Source: CAD feature listing. Evaluate the final solid. Frame: model axes, mm. A direction names the side the tool comes from. Coordinates: 2 decimals unless noted, no trailing zeros. Write each loop counter-clockwise with the first axis right and the second up, starting at its lowest first coordinate (ties: lowest second). Pieces come first, ordered by that corner, then holes. Notation, with made-up numbers: (11.25, 86.5) -> (25.25, 86.5) arc R9 cw to (25.25, 101.5) -> close; hole circle Ø4 at (46.25, 11). An arc over 180 degrees is marked (long way). Write item = value, one per line.
from build123d import *

# Parameters (mm, degrees)
SKETCH1_W           = 540
SKETCH1_H           = 330
BOSS_EXTRUDE1_DEPTH = 3
SKETCH2_W           = 540
SKETCH2_H           = 330
SKETCH2_W_2         = 500
SKETCH2_H_2         = 290
BOSS_EXTRUDE2_DEPTH = 25
FILLET1_R           = 5
SKETCH4_R           = 1.6
CUT_EXTRUDE1_DEPTH  = 28
SKETCH5_R           = 15
CUT_EXTRUDE2_DEPTH  = 3
SKETCH6_W           = 10
SKETCH6_H           = 290
BOSS_EXTRUDE3_DEPTH = 10
FILLET3_R           = 4
CHAMFER1_SIZE       = 5
SKETCH7_R           = 2.6
CUT_EXTRUDE3_DEPTH  = 3
SKETCH9_R           = 2.6
CUT_EXTRUDE4_DEPTH  = 47
SKETCH11_W          = 8
SKETCH11_H          = 140
BOSS_EXTRUDE4_DEPTH = 66
SKETCH12_R          = 6.1
CUT_EXTRUDE5_DEPTH  = 8
SKETCH13_W          = 8
SKETCH13_H          = 69
SKETCH13_W_2        = 20
SKETCH13_H_2        = 40.75
BOSS_EXTRUDE5_DEPTH = 27
SKETCH15_W          = 8
SKETCH15_H          = 47
CUT_EXTRUDE6_DEPTH  = 66
FILLET4_R           = 4
FILLET5_R           = 10
FILLET6_R           = 5
FILLET7_R           = 5
CHAMFER2_SIZE       = 5


with BuildPart() as part:
    # Sketch1 → Boss-Extrude1 (new body)
    with BuildSketch(Plane(origin=(0, 0, 0), x_dir=(1, 0, 0), z_dir=(0, 1, 0))):
        Rectangle(SKETCH1_W, SKETCH1_H)
    extrude(amount=BOSS_EXTRUDE1_DEPTH)

    # Sketch2 → Boss-Extrude2 (add)
    with BuildSketch(Plane(origin=(0, 3, 0), x_dir=(1, 0, 0), z_dir=(0, 1, 0))):
        Rectangle(SKETCH2_W, SKETCH2_H)
        Rectangle(SKETCH2_W_2, SKETCH2_H_2, mode=Mode.SUBTRACT)
    extrude(amount=BOSS_EXTRUDE2_DEPTH)

    # Fillet1
    fillet1_edges = [part.edges().sort_by_distance(p)[0] for p in [
        (270, 14, 165),
        (-270, 14, 165),
        (-270, 14, -165),
        (270, 14, -165),
    ]]
    fillet(fillet1_edges, radius=FILLET1_R)

    # Sketch4 → Cut-Extrude1 (cut)
    with BuildSketch(Plane(origin=(0, 28, 0), x_dir=(1, 0, 0), z_dir=(0, 1, 0))):
        with Locations(Location((-264, 120, 0), (0, 0, 270))):
            Circle(SKETCH4_R)
        with Locations(Location((-264, 40, 0), (0, 0, 270))):
            Circle(SKETCH4_R)
        with Locations(Location((-210, 159, 0), (0, 0, 270))):
            Circle(SKETCH4_R)
        with Locations(Location((-130, 159, 0), (0, 0, 270))):
            Circle(SKETCH4_R)
        with Locations(Location((-50, 159, 0), (0, 0, 270))):
            Circle(SKETCH4_R)
        with Locations(Location((50, 159, 0), (0, 0, 90))):
            Circle(SKETCH4_R)
        with Locations(Location((130, 159, 0), (0, 0, 90))):
            Circle(SKETCH4_R)
        with Locations(Location((210, 159, 0), (0, 0, 90))):
            Circle(SKETCH4_R)
        with Locations(Location((264, 40, 0), (0, 0, 90))):
            Circle(SKETCH4_R)
        with Locations(Location((264, 120, 0), (0, 0, 90))):
            Circle(SKETCH4_R)
    extrude(amount=-CUT_EXTRUDE1_DEPTH, mode=Mode.SUBTRACT)

    # Sketch5 → Cut-Extrude2 (cut)
    with BuildSketch(Plane(origin=(0, 3, 0), x_dir=(1, 0, 0), z_dir=(0, 1, 0))):
        with Locations(Location((0, 0, 0), (0, 0, 270))):
            Circle(SKETCH5_R)
    extrude(amount=-CUT_EXTRUDE2_DEPTH, mode=Mode.SUBTRACT)

    # Sketch6 → Boss-Extrude3 (add)
    with BuildSketch(Plane(origin=(0, 3, 0), x_dir=(1, 0, 0), z_dir=(0, 1, 0))):
        with Locations((25, 0)):
            Rectangle(SKETCH6_W, SKETCH6_H)
        with Locations((-25, 0)):
            Rectangle(SKETCH6_W, SKETCH6_H)
    extrude(amount=BOSS_EXTRUDE3_DEPTH)

    # Fillet3
    fillet3_edges = [part.edges().sort_by_distance(p)[0] for p in [
        (30, 3, 0),
        (30, 8, 145),
        (30, 8, -145),
        (20, 3, 0),
        (20, 8, -145),
        (20, 8, 145),
        (30, 13, 0),
        (25, 13, -145),
        (20, 13, 0),
        (25, 13, 145),
        (-20, 3, 0),
        (-20, 8, 145),
        (-20, 8, -145),
        (-30, 3, 0),
        (-30, 8, -145),
        (-30, 8, 145),
        (-20, 13, 0),
        (-25, 13, -145),
        (-30, 13, 0),
        (-25, 13, 145),
    ]]
    fillet(fillet3_edges, radius=FILLET3_R)

    # Chamfer1
    # the kernel refuses this chamfer: 5 mm, written as the material it takes off along each edge
    with BuildSketch(Plane(origin=(-270, 0, -160), x_dir=(0, 1, 0), z_dir=(0, 0, 1)), Plane(origin=(270, 0, 160), x_dir=(0, 1, 0), z_dir=(0, 0, -1))) as chamfer1_piece_1:
        Polygon((CHAMFER1_SIZE, 0), (0, -CHAMFER1_SIZE), (0, 0), align=None)
    extrude(amount=320, mode=Mode.SUBTRACT)
    with BuildSketch(Plane(origin=(-265, 0, 165), x_dir=(0, 1, 0), z_dir=(1, 0, 0)), Plane(origin=(265, 0, -165), x_dir=(0, 1, 0), z_dir=(-1, 0, 0))) as chamfer1_piece_2:
        Polygon((CHAMFER1_SIZE, 0), (0, -CHAMFER1_SIZE), (0, 0), align=None)
    extrude(amount=530, mode=Mode.SUBTRACT)
    with BuildSketch(Plane(origin=(265, 0, -160), x_dir=(0, 0, -1), z_dir=(-1, 0, 0))) as chamfer1_piece_3:
        Polygon((5, -CHAMFER1_SIZE), (5 - CHAMFER1_SIZE, 0), (5, 0), align=None)
    revolve(axis=Axis((265, 0, -160), (0, -1, 0)), revolution_arc=90, mode=Mode.SUBTRACT)
    with BuildSketch(Plane(origin=(265, 0, 160), x_dir=(0, 0, 1), z_dir=(-1, 0, 0))) as chamfer1_piece_4:
        Polygon((5, CHAMFER1_SIZE), (5 - CHAMFER1_SIZE, 0), (5, 0), align=None)
    revolve(axis=Axis((265, 0, 160), (0, 1, 0)), revolution_arc=90, mode=Mode.SUBTRACT)
    with BuildSketch(Plane(origin=(-265, 0, 160), x_dir=(0, 0, 1), z_dir=(1, 0, 0))) as chamfer1_piece_5:
        Polygon((5, -CHAMFER1_SIZE), (5 - CHAMFER1_SIZE, 0), (5, 0), align=None)
    revolve(axis=Axis((-265, 0, 160), (0, -1, 0)), revolution_arc=90, mode=Mode.SUBTRACT)
    with BuildSketch(Plane(origin=(-265, 0, -160), x_dir=(0, 0, -1), z_dir=(1, 0, 0))) as chamfer1_piece_6:
        Polygon((5, CHAMFER1_SIZE), (5 - CHAMFER1_SIZE, 0), (5, 0), align=None)
    revolve(axis=Axis((-265, 0, -160), (0, 1, 0)), revolution_arc=90, mode=Mode.SUBTRACT)

    # Sketch7 → Cut-Extrude3 (cut)
    with BuildSketch(Plane.XZ):
        with Locations(Location((-60, 60, 0), (0, 0, 270))):
            Circle(SKETCH7_R)
        with Locations(Location((60, 60, 0), (0, 0, 270))):
            Circle(SKETCH7_R)
        with Locations(Location((60, -60, 0), (0, 0, 270))):
            Circle(SKETCH7_R)
        with Locations(Location((-60, -60, 0), (0, 0, 270))):
            Circle(SKETCH7_R)
    extrude(amount=-CUT_EXTRUDE3_DEPTH, mode=Mode.SUBTRACT)

    # Sketch9 → Cut-Extrude4 (cut)
    with BuildSketch(Plane.XZ):
        with Locations(Location((-38.890872965, 38.890872965, 0), (0, 0, 270))):
            Circle(SKETCH9_R)
        with Locations(Location((38.890872965, 38.890872965, 0), (0, 0, 270))):
            Circle(SKETCH9_R)
        with Locations(Location((38.890872965, -38.890872965, 0), (0, 0, 270))):
            Circle(SKETCH9_R)
        with Locations(Location((-38.890872965, -38.890872965, 0), (0, 0, 270))):
            Circle(SKETCH9_R)
    extrude(amount=-CUT_EXTRUDE4_DEPTH, mode=Mode.SUBTRACT)

    # Sketch11 → Boss-Extrude4 (add)
    with BuildSketch(Plane(origin=(0, 3, 0), x_dir=(1, 0, 0), z_dir=(0, 1, 0))):
        with Locations((-219, 0)):
            Rectangle(SKETCH11_W, SKETCH11_H)
    extrude(amount=BOSS_EXTRUDE4_DEPTH)

    # Sketch12 → Cut-Extrude5 (cut)
    with BuildSketch(Plane.ZY.offset(223)):
        with Locations((0, 53)):
            Circle(SKETCH12_R)
    extrude(amount=-CUT_EXTRUDE5_DEPTH, mode=Mode.SUBTRACT)

    # Sketch13 → Boss-Extrude5 (add)
    with BuildSketch(Plane.ZY.offset(223)):
        with Locations((19, 34.5)):
            Rectangle(SKETCH13_W, SKETCH13_H)
        with Locations((-60, 20.375)):
            Rectangle(SKETCH13_W_2, SKETCH13_H_2)
    extrude(amount=BOSS_EXTRUDE5_DEPTH)

    # Sketch15 → Cut-Extrude6 (cut)
    with BuildSketch(Plane(origin=(0, 69, 0), x_dir=(1, 0, 0), z_dir=(0, 1, 0))):
        with Locations((-219, -46.5)):
            Rectangle(SKETCH15_W, SKETCH15_H)
    extrude(amount=-CUT_EXTRUDE6_DEPTH, mode=Mode.SUBTRACT)

    # Fillet4
    fillet4_edges = [part.edges().sort_by_distance(p)[0] for p in [
        (-232.5, 3, -70),
        (-232.5, 3, 23),
        (-215, 3, -23.5),
        (-215, 36, 23),
    ]]
    fillet(fillet4_edges, radius=FILLET4_R)

    # Fillet5
    fillet5_edges = [part.edges().sort_by_distance(p)[0] for p in [
        (-223, 40.75, -60),
    ]]
    fillet(fillet5_edges, radius=FILLET5_R)

    # Fillet6
    fillet6_edges = [part.edges().sort_by_distance(p)[0] for p in [
        (-250, 40.75, -60),
    ]]
    fillet(fillet6_edges, radius=FILLET6_R)

    # Fillet7
    fillet7_edges = [part.edges().sort_by_distance(p)[0] for p in [
        (-219, 69, -70),
    ]]
    fillet(fillet7_edges, radius=FILLET7_R)

    # Chamfer2
    chamfer2_edges = [part.edges().sort_by_distance(p)[0] for p in [
        (-215, 53, -6.1),
    ]]
    chamfer(chamfer2_edges, length=CHAMFER2_SIZE)


solid = part.part
1) Cut plane B-B, the plane x = -171. Output: boundary loops of the cut face in (y, z).
Answer block:
outline = (0, -160) -> (5, -165) -> (28, -165) -> (28, -145) -> (3, -145) -> (3, 145) -> (28, 145) -> (28, 165) -> (5, 165) -> (0, 160) -> close
2) Material intervals for probe 1 along X at (y, z) = (15.5, -36); probe 2 along Z at (x, y) = (264, 15); probe 3 along X at (y, z) = (16, -120), sorted ascending. Write a range as [from, to].
Answer block:
probe_1 = [-270, -250], [-223, -215], [250, 270]
probe_2 = [-165, -121.6], [-118.4, -41.6], [-38.4, 165]
probe_3 = [-270, -265.6], [-262.4, -250], [250, 262.4], [265.6, 270]
3) Pull-direction query (Z, two-part tool) for faces 1 (the flat face through (-250, 15, 85)), 2 (the flat face through (-4, 16, -165)), 3 (the flat face through (-21, 28, 146)); classes: +Z half, -Z half, draft (parallel to the pull), parting line (faces both ways), or undercut.
Answer block:
face_1 = undercut
face_2 = -Z half
face_3 = draft
4) Cut plane D-D, the plane z = -104. Output: boundary loops of the cut face in (x, y), and give its area (4 significant figures).
Answer block:
outline = (-270, 5) -> (-265, 0) -> (265, 0) -> (270, 5) -> (270, 28) -> (250, 28) -> (250, 3) -> (34, 3) arc R4 cw to (30, 7) -> (30, 9) arc R4 ccw to (26, 13) -> (24, 13) arc R4 ccw to (20, 9) -> (20, 7) arc R4 cw to (16, 3) -> (-16, 3) arc R4 cw to (-20, 7) -> (-20, 9) arc R4 ccw to (-24, 13) -> (-26, 13) arc R4 ccw to (-30, 9) -> (-30, 7) arc R4 cw to (-34, 3) -> (-250, 3) -> (-250, 28) -> (-270, 28) -> close
area = 2,795 mm2
5) Reachability of faces 4 (the cylindrical face through (-225.85, 43.76, -59.86)), 5 (the flat face through (-236, 36, 15)), 6 (the cylindrical face through (-221.521, 47.045, -1.322)) from +Z, -Z, +X, -X, +Y, -Y: full face, straight path, thin tool, end or side. Return the list, or none.
Answer block:
face_4 = -Z, -X, +Y
face_5 = +Y
face_6 = +X, -X
6) Cut plane A-A, the plane x = 0. Output: boundary loops of the cut face in (y, z).
Answer block:
outline = (0, -160) -> (5, -165) -> (28, -165) -> (28, -145) -> (3, -145) -> (3, -15) -> (0, -15) -> close; (0, 15) -> (3, 15) -> (3, 145) -> (28, 145) -> (28, 165) -> (5, 165) -> (0, 160) -> close
7) Cut plane C-C, the plane z = 0. Give the number of separate pieces and of enclosed holes in the cut face, and give its area (3 significant figures).
Answer block:
separate_pieces = 3
enclosed_holes = 0
area = 3,110 mm2
8) First-contact query: pin 1 Ø5 at (x, z) = (7.5, 49.5) entering from +Y; pin 2 Ø3.5 at (x, z) = (264, -120) entering from +Y; pin 3 Ø1.6 at (x, z) = (25, 44) entering from +Y; pin 4 Ø8.5 at (y, z) = (32, -58) entering from -X. Flat tips, straight axial feed; report the tip coordinate or a pass-through.
Answer block:
pin_1 = 3
pin_2 = 28
pin_3 = 13
pin_4 = -270
